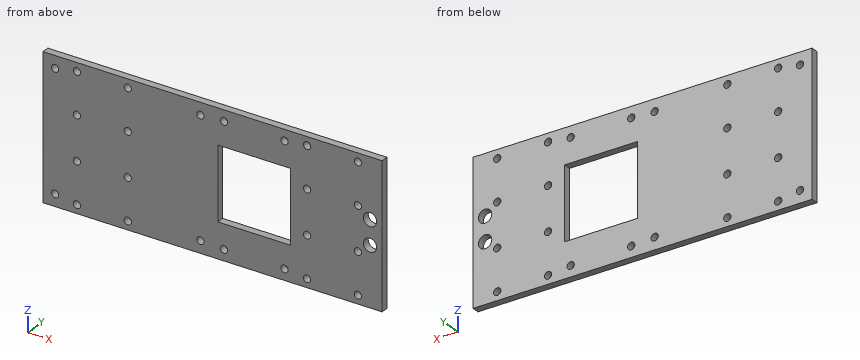
from build123d import *

# Parameters (mm, degrees)
SKETCH1_W           = 140
SKETCH1_H           = 59
SKETCH1_R           = 1.5
SKETCH1_W_2         = 30
SKETCH1_H_2         = 30
BOSS_EXTRUDE1_DEPTH = 3
SKETCH8_R           = 2.75
CUT_EXTRUDE6_DEPTH  = 77.021378572


with BuildPart() as part:
    # Sketch1 → Boss-Extrude1 (new body)
    with BuildSketch(Plane(origin=(0, 0, 0), x_dir=(1, 0, 0), z_dir=(0, 1, 0))):
        Rectangle(SKETCH1_W, SKETCH1_H)
        with Locations(Location((-35, 26, 0), (0, 0, 270))):
            Circle(SKETCH1_R, mode=Mode.SUBTRACT)
        with Locations(Location((-56, 26, 0), (0, 0, 270))):
            Circle(SKETCH1_R, mode=Mode.SUBTRACT)
        with Locations(Location((-56, 9, 0), (0, 0, 270))):
            Circle(SKETCH1_R, mode=Mode.SUBTRACT)
        with Locations(Location((-35, 9, 0), (0, 0, 270))):
            Circle(SKETCH1_R, mode=Mode.SUBTRACT)
        with Locations(Location((-35, -9, 0), (0, 0, 270))):
            Circle(SKETCH1_R, mode=Mode.SUBTRACT)
        with Locations(Location((-56, -9, 0), (0, 0, 270))):
            Circle(SKETCH1_R, mode=Mode.SUBTRACT)
        with Locations(Location((-35, -26, 0), (0, 0, 270))):
            Circle(SKETCH1_R, mode=Mode.SUBTRACT)
        with Locations(Location((-56, -26, 0), (0, 0, 270))):
            Circle(SKETCH1_R, mode=Mode.SUBTRACT)
        with Locations(Location((60, 26, 0), (0, 0, 270))):
            Circle(SKETCH1_R, mode=Mode.SUBTRACT)
        with Locations(Location((39, 26, 0), (0, 0, 270))):
            Circle(SKETCH1_R, mode=Mode.SUBTRACT)
        with Locations(Location((39, -9, 0), (0, 0, 270))):
            Circle(SKETCH1_R, mode=Mode.SUBTRACT)
        with Locations(Location((60, -9, 0), (0, 0, 270))):
            Circle(SKETCH1_R, mode=Mode.SUBTRACT)
        with Locations(Location((60, -26, 0), (0, 0, 270))):
            Circle(SKETCH1_R, mode=Mode.SUBTRACT)
        with Locations(Location((39, -26, 0), (0, 0, 270))):
            Circle(SKETCH1_R, mode=Mode.SUBTRACT)
        with Locations(Location((60, 9, 0), (0, 0, 270))):
            Circle(SKETCH1_R, mode=Mode.SUBTRACT)
        with Locations(Location((39, 9, 0), (0, 0, 270))):
            Circle(SKETCH1_R, mode=Mode.SUBTRACT)
        with Locations(Location((-5, -24.5, 0), (0, 0, 270))):
            Circle(SKETCH1_R, mode=Mode.SUBTRACT)
        with Locations(Location((-5, 24.5, 0), (0, 0, 270))):
            Circle(SKETCH1_R, mode=Mode.SUBTRACT)
        with Locations(Location((-65, 24.5, 0), (0, 0, 270))):
            Circle(SKETCH1_R, mode=Mode.SUBTRACT)
        with Locations(Location((-65, -24.5, 0), (0, 0, 270))):
            Circle(SKETCH1_R, mode=Mode.SUBTRACT)
        with Locations(Location((29.671375392, 25, 0), (0, 0, 270))):
            Circle(SKETCH1_R, mode=Mode.SUBTRACT)
        with Locations(Location((29.671375392, -25, 0), (0, 0, 270))):
            Circle(SKETCH1_R, mode=Mode.SUBTRACT)
        with Locations(Location((4.671375392, -25, 0), (0, 0, 270))):
            Circle(SKETCH1_R, mode=Mode.SUBTRACT)
        with Locations(Location((4.671375392, 25, 0), (0, 0, 270))):
            Circle(SKETCH1_R, mode=Mode.SUBTRACT)
        with Locations((17.171375392, 0)):
            Rectangle(SKETCH1_W_2, SKETCH1_H_2, mode=Mode.SUBTRACT)
    extrude(amount=BOSS_EXTRUDE1_DEPTH)

    # Sketch8 → Cut-Extrude6 (cut, through all)
    with BuildSketch(Plane(origin=(0, 3, 0), x_dir=(1, 0, 0), z_dir=(0, 1, 0))):
        with Locations(Location((65, 5, 0), (0, 0, 270))):
            Circle(SKETCH8_R)
        with Locations(Location((65, -5, 0), (0, 0, 270))):
            Circle(SKETCH8_R)
    extrude(amount=-CUT_EXTRUDE6_DEPTH, mode=Mode.SUBTRACT)


solid = part.part
Input: part model. Units: mm. Frame: model coordinates. Give positions to 0.01 mm unless a question says otherwise; leave off trailing zeros. Write each loop counter-clockwise with the first axis right and the second up, starting at its lowest first coordinate (ties: lowest second). Pieces come first, ordered by that corner, then holes. Notation, with made-up numbers: M -36.75,0 L 7.25,0 A34 cw 7.25,30 Z; hole C 45,30 d2. An arc over 180 degrees is marked long. Write item = value, one per line. Start each with the question number.
1) Material intervals for line 1 along X through (y, z) = (1.3, 5); line 2 along X through (y, z) = (1, 9); line 3 along X through (y, z) = (0.7, 0), sorted ascending. Write a range as [from, to].
2) Cut plane B-B on x = -35. Return the cut outline in (y, z), then the cut area to 3 significant figures.
3) Cut plane D-D on x = 20. Return the cut outline in (y, z), then the cut area to 3 significant figures.
4) Cut plane A-A on z = -13. Return the cut outline in (x, y), then the cut area to 3 significant figures.
5) Cut plane C-C on z = 9. Return the cut outline in (x, y), then the cut area to 3 significant figures.
6) First-contact query: pin 1 Ø1.8 at (x, z) = (4.67, 25) entering from -Y. Flat tip, straight axial feed; report the tip coordinate or a pass-through.
Solved:
q1.line_1 = [-70, 2.17], [32.17, 62.25], [67.75, 70]
q1.line_2 = [-70, -57.5], [-54.5, -36.5], [-33.5, 2.17], [32.17, 37.5], [40.5, 58.5], [61.5, 70]
q1.line_3 = [-70, 2.17], [32.17, 70]
q2.outline = M 0,-29.5 L 3,-29.5 L 3,-27.5 L 0,-27.5 Z; M 0,-24.5 L 3,-24.5 L 3,-10.5 L 0,-10.5 Z; M 0,-7.5 L 3,-7.5 L 3,7.5 L 0,7.5 Z; M 0,10.5 L 3,10.5 L 3,24.5 L 0,24.5 Z; M 0,27.5 L 3,27.5 L 3,29.5 L 0,29.5 Z
q2.area = 141 mm2
q3.outline = M 0,-29.5 L 3,-29.5 L 3,-15 L 0,-15 Z; M 0,15 L 3,15 L 3,29.5 L 0,29.5 Z
q3.area = 87.0 mm2
q4.outline = M -70,0 L 2.17,0 L 2.17,3 L -70,3 Z; M 32.17,0 L 70,0 L 70,3 L 32.17,3 Z
q4.area = 330 mm2
q5.outline = M -70,0 L -57.5,0 L -57.5,3 L -70,3 Z; M -54.5,0 L -36.5,0 L -36.5,3 L -54.5,3 Z; M -33.5,0 L 2.17,0 L 2.17,3 L -33.5,3 Z; M 32.17,0 L 37.5,0 L 37.5,3 L 32.17,3 Z; M 40.5,0 L 58.5,0 L 58.5,3 L 40.5,3 Z; M 61.5,0 L 70,0 L 70,3 L 61.5,3 Z
q5.area = 294 mm2
q6.pin_1 = through
